Can you work these out from the model? Positions are in its coordinate system, mm. A direction names the side the tool comes from. Coordinates: 2 decimals unless noted, no trailing zeros. Order: outer loops, then holes, each group sorted by start corner. A loop starts at its lowest first (then second) coordinate and runs counter-clockwise, first axis right, second up. Notation, with made-up numbers: (75.25, 50.25) -> (99.25, 50.25) arc R23 ccw to (99.25, 87.25) -> close; hole circle Ø2 at (51.25, 34). An arc over 180 degrees is marked (long way). Answer in a Markdown table with one row per item.
```python
from build123d import *

# Parameters (mm, degrees)
F0_W     = 3.556
F0_H     = 3.302
F0_W_2   = 4.572
F0_H_2   = 72.771
F0_W_3   = 15.24
F1_DEPTH = 609.6
F2_R     = 5.08


with BuildPart() as f1:
    # F0 (on Front) → F1 (new body)
    with BuildSketch(Plane.XZ):
        with Locations((-1.778, 1.651)):
            Rectangle(F0_W, F0_H)
        with Locations((-5.842, 1.651)):
            Rectangle(F0_W_2, F0_H)
        with Locations((-1.778, 39.6875)):
            Rectangle(F0_W, F0_H_2)
        with Locations((-1.778, 77.724)):
            Rectangle(F0_W, F0_H)
        with Locations((-11.176, 77.724)):
            Rectangle(F0_W_3, F0_H)
    extrude(amount=F1_DEPTH)

    # F2
    f2_edges = [f1.edges().sort_by_distance(p)[0] for p in [
        (0, -304.8, 79.375),
        (0, -304.8, 0),
    ]]
    fillet(f2_edges, radius=F2_R)


solid = f1.part
```
(1) Suppose I cut it at B-B (z = 42.5). Please give me the cut outline in (x, y), and give its area (3 significant figures).
Response values:
| item | result |
|---|---|
| outline | (-3.56, -609.6) -> (0, -609.6) -> (0, 0) -> (-3.56, 0) -> close |
| area | 2,170 mm2 |
(2) We'd pull the mould along Z, two halves only. Please class faces 3 (the flat face through (-1, -609.6, 43)), 4 (the flat face through (-11, -301, 76.073)), 5 (the flat face through (-12, -301, 79.375)): +Z half, -Z half, draft (parallel to the pull), parting line (faces both ways), or undercut.
Response values:
| item | result |
|---|---|
| face 3 | draft |
| face 4 | undercut |
| face 5 | +Z half |
(3) Suppose I cut it at A-A (y = -523). Please give me the cut outline in (x, z) (3 decimals).
Response values:
| item | result |
|---|---|
| outline | (-18.796, 76.073) -> (-3.556, 76.073) -> (-3.556, 3.302) -> (-8.128, 3.302) -> (-8.128, 0) -> (-5.08, 0) arc R5.08 ccw to (0, 5.08) -> (0, 74.295) arc R5.08 ccw to (-5.08, 79.375) -> (-18.796, 79.375) -> close |
(4) I need wall thicknesses on line 1 (Z direction, x = -6.5, y = -159) (3 decimals); line 2 (Z direction, x = -4.5, y = -571.5); line 3 (X direction, y = -533, z = 74.5). Which ranges of each line are inside material? Lowest first, please. Write a range as [from, to].
Response values:
| item | result |
|---|---|
| line 1 | [0, 3.302], [76.073, 79.375] |
| line 2 | [0.03, 3.3], [76.07, 79.34] |
| line 3 | [-3.56, 0] |
(5) Suppose I cut it at C-C (x = -13.5). Please give me the cut outline in (y, z) (3 decimals), and give its area (3 significant figures).
Response values:
| item | result |
|---|---|
| outline | (-609.6, 76.073) -> (0, 76.073) -> (0, 79.375) -> (-609.6, 79.375) -> close |
| area | 2,010 mm2 |
(6) Will these pins go through, and if not, where does the flat tip stop? pin 1 Ø3.5 at (y, z) = (-413, 2.5) entering from -X; pin 2 Ø3 at (y, z) = (-545, 11) entering from -X.
Response values:
| item | result |
|---|---|
| pin 1 | x = -8.13 |
| pin 2 | x = -3.56 |
(7) On a 3-axis mill with a long thin cutter (end or side, diameter ignored), from which of +Z, -Z, +X, -X, +Y, -Y can I reach the whole of each face in a straight line? I mean faces 1 (the flat face through (-3.556, -301, 40)), 2 (the flat face through (-1, 0, 43)). Say none if no direction works.
Response values:
| item | result |
|---|---|
| face 1 | -X, +Y, -Y |
| face 2 | +Z, -Z, +X, -X, +Y |
